Check sheet for the drawn part. Datum: minimum x, y, z corner. Units: mm. A direction names the side the tool comes from. Round coordinates to 2 decimals unless told otherwise and drop trailing zeros. Order: outer loops, then holes, each group sorted by start corner. A loop starts at its lowest first (then second) coordinate and runs counter-clockwise, first axis right, second up. Notation, with made-up numbers: (54.5, 27) -> (72.5, 27) arc R24 cw to (72.5, 66) -> close; hole circle Ø5 at (29.25, 57). An arc over 180 degrees is marked (long way). Answer as a JSON object with one key per item and string values. Group by question number.
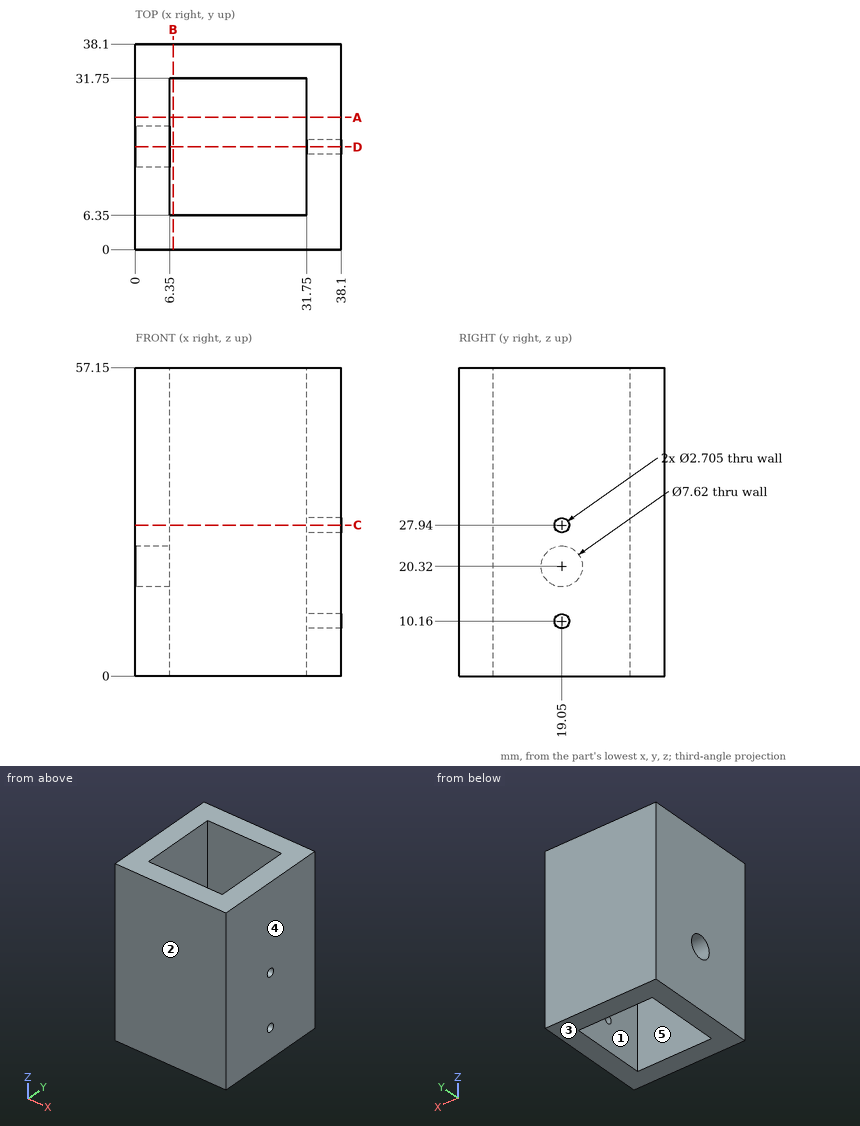
Item 1: Depth check by flat-ended pin: pin 1 Ø2 at (y, z) = (19.05, 27.94) entering from +X. Enter the tip coordinate at first touch or a pass-through.
Item 2: Sectioned sample at D-D, the plane y = 19.05. Enter the section's corners in (x, z), then the cut area to 3 significant figures.
Item 3: Thickness scan on L1, parallel to Y at x = 14, z = 48.5; L2, parallel to Z at x = 33, y = 19. Record the ranges inside material, lowest first.
Item 4: Set-up check for the marked faces 4 and 5: record each of +Z, -Z, +X, -X, +Y, -Y from which the full face is reachable in a straight line by a thin tool's end or side.
Item 5: Sectioned sample at A-A, the plane y = 24.5. Enter the section's corners in (x, z).
Item 6: Mould release check, pull along Y, two halves, no side actions. Record for the marked faces 1, 2 and 3: pulls with the +Y half, pulls with the -Y half, needs draft (parallel to the pull), parting line crosses it, or undercut.
Item 7: Sectioned sample at C-C, the plane z = 27.94. Enter the section's corners in (x, y), then the cut area to 3 significant figures.
Result:
{
 "1": {"pin 1": "stops at x = 6.35"},
 "2": {"outline": "(0, 0) -> (6.35, 0) -> (6.35, 16.51) -> (0, 16.51) -> close; (0, 24.13) -> (6.35, 24.13) -> (6.35, 57.15) -> (0, 57.15) -> close; (31.75, 0) -> (38.1, 0) -> (38.1, 8.81) -> (31.75, 8.81) -> close; (31.75, 11.51) -> (38.1, 11.51) -> (38.1, 26.59) -> (31.75, 26.59) -> close; (31.75, 29.29) -> (38.1, 29.29) -> (38.1, 57.15) -> (31.75, 57.15) -> close", "area": "643 mm2"},
 "3": {"L1": "y = 0 to 6.35, 31.75 to 38.1", "L2": "z = 0 to 8.81, 11.51 to 26.59, 29.29 to 57.15"},
 "4": {"face 4": "+Z, -Z, +X, +Y, -Y", "face 5": "+Z, -Z"},
 "5": {"outline": "(0, 0) -> (6.35, 0) -> (6.35, 57.15) -> (0, 57.15) -> close; (31.75, 0) -> (38.1, 0) -> (38.1, 57.15) -> (31.75, 57.15) -> close"},
 "6": {"face 1": "undercut", "face 2": "pulls with the -Y half", "face 3": "needs draft"},
 "7": {"outline": "(0, 0) -> (38.1, 0) -> (38.1, 17.7) -> (31.75, 17.7) -> (31.75, 6.35) -> (6.35, 6.35) -> (6.35, 31.75) -> (31.75, 31.75) -> (31.75, 20.4) -> (38.1, 20.4) -> (38.1, 38.1) -> (0, 38.1) -> close", "area": "789 mm2"}
}
